For this review, take the finished solid that the model builds, in its own axes (mm). Give positions to 0.01 mm unless a question says otherwise; leave off trailing zeros. Order: outer loops, then holes, each group sorted by start corner. A loop starts at its lowest first (then second) coordinate and runs counter-clockwise, first axis right, second up.
Autodesk Inventor part; units mm, degrees
ref_plane "YZ Plane" through (0, 0, 0) normal (1, 0, 0) x (0, 1, 0)
ref_plane "XZ Plane" through (0, 0, 0) normal (0, 1, 0) x (-1, 0, 0)
ref_plane "XY Plane" through (0, 0, 0) normal (0, 0, 1) x (1, 0, 0)
sketch "Sketch1" plane through (0, 0, 0) normal (0, 0, 1) x (1, 0, 0)
  line L0 (-204.47, 0) -> (204.47, 0)
  line L1 (0, -204.47) -> (0, 204.47)
  circle A0 centre (0, 0) radius 146.05
  dimension "d0" = 292.1
extrude "Extrusion1" add sketch "Sketch1" along normal blind 6
sketch "Sketch2" plane through (0, 0, 6) normal (0, 0, 1) x (1, 0, 0)
  circle A0 centre (0, 0) radius 114.3 construction
  arc A1 (-1.4999, 88.8873) -> (1.4999, 88.8873) centre (0, 0) ccw construction
  line L0 (-204.47, 0) -> (204.47, 0) construction
  line L1 (0, -204.47) -> (0, 204.47) construction
  arc A2 (1.4999, 114.2873) -> (-1.5, 114.2902) centre (0, 114.3) ccw
  arc A3 (-1.5, 88.9098) -> (1.4999, 88.9127) centre (0, 88.9) ccw
  line L2 (1.4999, 114.2902) -> (1.4999, 88.8873)
  line L3 (-1.5, 88.8873) -> (-1.5, 114.2902)
  arc A4 (-114.2873, 1.4999) -> (-114.2902, -1.5) centre (-114.3, 0) ccw
  arc A5 (-88.9098, -1.5) -> (-88.9127, 1.4999) centre (-88.9, 0) ccw
  line L4 (-114.2902, 1.4999) -> (-88.8873, 1.4999)
  line L5 (-88.8873, -1.5) -> (-114.2902, -1.5)
  arc A6 (-1.4999, -114.2873) -> (1.5, -114.2902) centre (0, -114.3) ccw
  arc A7 (1.5, -88.9098) -> (-1.4999, -88.9127) centre (0, -88.9) ccw
  line L6 (-1.4999, -114.2902) -> (-1.4999, -88.8873)
  line L7 (1.5, -88.8873) -> (1.5, -114.2902)
  arc A8 (88.9098, 1.5) -> (88.9127, -1.4999) centre (88.9, 0) ccw
  line L8 (88.8873, 1.5) -> (114.2902, 1.5)
  arc A9 (114.2873, -1.4999) -> (114.2902, 1.5) centre (114.3, 0) ccw
  line L9 (114.2902, -1.4999) -> (88.8873, -1.4999)
  point P0 (-88.8873, -1.4999)
  point P1 (1.4999, -88.8873)
  point P2 (88.8873, 1.4999)
  dimension "d3" = 228.6
  dimension "d4" = 177.8
  dimension "d5" = 3
  dimension "d6" = 3
  dimension "d13" = 3
  dimension "d14" = 3
  dimension "d15" = 3
  dimension "d16" = 3
  dimension "d17" = 3
  dimension "d18" = 3
extrude "Extrusion2" cut sketch "Sketch2" against normal blind 6
sketch "Sketch4" plane through (0, 0, 6) normal (0, 0, 1) x (1, 0, 0)
  line L0 (-204.47, 0) -> (204.47, 0)
  line L1 (0, -204.47) -> (0, 204.47)
  line L2 (-17, 70) -> (-15, 70)
  line L3 (-15, 70) -> (-15, 50)
  line L4 (-15, 50) -> (-17, 50)
  line L5 (-17, 50) -> (-17, 70)
  line L6 (17, 70) -> (15, 70)
  line L7 (15, 70) -> (15, 50)
  line L8 (15, 50) -> (17, 50)
  line L9 (17, 50) -> (17, 70)
  line L10 (-17, -70) -> (-15, -70)
  line L11 (-15, -70) -> (-15, -50)
  line L12 (-15, -50) -> (-17, -50)
  line L13 (-17, -50) -> (-17, -70)
  line L14 (17, -70) -> (15, -70)
  line L15 (15, -70) -> (15, -50)
  line L16 (15, -50) -> (17, -50)
  line L17 (17, -50) -> (17, -70)
  line L18 (-70, -17) -> (-70, -15)
  line L19 (-70, -15) -> (-50, -15)
  line L20 (-50, -15) -> (-50, -17)
  line L21 (-50, -17) -> (-70, -17)
  line L22 (-70, 17) -> (-70, 15)
  line L23 (-70, 15) -> (-50, 15)
  line L24 (-50, 15) -> (-50, 17)
  line L25 (-50, 17) -> (-70, 17)
  line L26 (70, -17) -> (70, -15)
  line L27 (70, -15) -> (50, -15)
  line L28 (50, -15) -> (50, -17)
  line L29 (50, -17) -> (70, -17)
  line L30 (70, 17) -> (70, 15)
  line L31 (70, 15) -> (50, 15)
  line L32 (50, 15) -> (50, 17)
  line L33 (50, 17) -> (70, 17)
  point P0 (0, 0)
  dimension "d21" = 2
  dimension "d22" = 50
  dimension "d23" = 20
  dimension "d24" = 15
  dimension "d25" = 2
  dimension "d26" = 20
extrude "Extrusion3" cut sketch "Sketch4" against normal blind 6
sketch "Sketch5" plane through (0, 0, 0) normal (0, 0, -1) x (-1, 0, 0)
  circle A0 centre (66, 24.11) radius 1.75
  circle A1 centre (54, 24.11) radius 1.75
  circle A2 centre (54.9574, -24.11) radius 1.75
  circle A3 centre (64.9809, -24.11) radius 1.75
  point P0 (0, 0)
extrude "Extrusion4" cut sketch "Sketch5" against normal blind 10
properties part number "BallBallerina_BasePlate_v1"
1) We need section C-C on z = 4.85. Count the separate pieces of the cut face and the enclosed holes in it, then the cut area to 3 significant figures.
Answer sheet:
separate pieces: 1
enclosed holes: 16
area: 66,300 mm2
2) We need section A-A on y = 60.5. Give the boundary of the cut face in (x, z), then the cut area to 3 significant figures.
Answer sheet:
outline: (-132.93, 0) - (-17, 0) - (-17, 6) - (-132.93, 6) - close; (-15, 0) - (15, 0) - (15, 6) - (-15, 6) - close; (17, 0) - (132.93, 0) - (132.93, 6) - (17, 6) - close
area: 1,570 mm2
3) We need section B-B on x = -95.5. Give the boundary of the cut face in (y, z), then the cut area to 3 significant figures.
Answer sheet:
outline: (-110.5, 0) - (-1.5, 0) - (-1.5, 6) - (-110.5, 6) - close; (1.5, 0) - (110.5, 0) - (110.5, 6) - (1.5, 6) - close
area: 1,310 mm2
4) We need section D-D on x = 110.5. Give the boundary of the cut face in (y, z), then the cut area to 3 significant figures.
Answer sheet:
outline: (-95.5, 0) - (-1.5, 0) - (-1.5, 6) - (-95.5, 6) - close; (1.5, 0) - (95.5, 0) - (95.5, 6) - (1.5, 6) - close
area: 1,130 mm2
5) Clearance check with flat-ended pins moving along their axes: pin 1 (0.6 mm diameter, centred on x = -16.5, z = 2, fed in from +Y); pin 2 (0.6 mm diameter, centred on y = -16.5, z = 2.5, fed in from -X); pin 3 (0.6 mm diameter, centred on y = 16.5, z = 3, fed in from +X); pin 4 (12 mm diameter, centred on x = -61.5, y = 19.5, fed in from -Z). State where each tip first meets the part, or that it passes through.
Answer sheet:
pin 1: stops at y = 145.15
pin 2: stops at x = -145.15
pin 3: stops at x = 145.15
pin 4: stops at z = 0
6) To check wall thickness, follow line 1 (Y direction, x = -58.5, z = 1.25); line 2 (Y direction, x = -66, z = 1.6); line 3 (Y direction, x = -54, z = 1.7). State the ranges of each line that lie inside material, in increasing order.
Answer sheet:
line 1: y = -133.82 to -17, -15 to 15, 17 to 133.82
line 2: y = -130.29 to -25.53, -22.69 to -17, -15 to 15, 17 to 22.36, 25.86 to 130.29
line 3: y = -135.7 to -25.57, -22.65 to -17, -15 to 15, 17 to 22.36, 25.86 to 135.7
